from build123d import *

# Parameters (mm, degrees)
BOSS_EXTRUDE1_START                = -3.2
BOSS_EXTRUDE1_DEPTH                = 3.2
SKETCH3_R                          = 2.4
BOSS_EXTRUDE2_DEPTH                = 9.2
SKETCH4_R                          = 2.4
BOSS_EXTRUDE3_DEPTH                = 1.2
BOSS_EXTRUDE3_TAPER                = 36
CUT_EXTRUDE1_DEPTH                 = 6.925
BOSS_EXTRUDE4_DEPTH                = 3.2
TAP_DRILL_FOR_M2_2_HELICOIL1_D     = 2.3
TAP_DRILL_FOR_M2_2_HELICOIL1_DEPTH = 9.2
TAP_DRILL_FOR_M2_2_HELICOIL1_TIP   = 0.690989712


with BuildPart() as part:
    # Sketch1 → Revolve1 (revolve)
    with BuildSketch(Plane.XY):
        with BuildLine():
            Line((1.985572965, 1.6), (4.15, 1.6))
            Line((4.15, 1.6), (4.15, -1.6))
            Line((4.15, -1.6), (1.985572965, -1.6))
            ThreePointArc((1.985572965, -1.6), (2.55, 0), (1.985572965, 1.6))
        make_face()
    revolve(axis=Axis((0, 0, 0), (0, 1, 0)))

    # Sketch2 → Boss-Extrude1 (add)
    with BuildSketch(Plane(origin=(0, 1.6, 0), x_dir=(1, 0, 0), z_dir=(0, 1, 0)).offset(BOSS_EXTRUDE1_START)):
        with BuildLine():
            Line((-2.4, -6.925), (-4.001507312, -1.100199632))
            ThreePointArc((-4.001507312, -1.100199632), (0, -4.15), (4.001507312, -1.100199632))
            Line((4.001507312, -1.100199632), (2.4, -6.925))
            Line((2.4, -6.925), (2.4, -13.85))
            Line((2.4, -13.85), (-2.4, -13.85))
            Line((-2.4, -13.85), (-2.4, -6.925))
        make_face()
    extrude(amount=BOSS_EXTRUDE1_DEPTH)

    # Sketch3 → Boss-Extrude2 (add)
    with BuildSketch(Plane.XY.offset(13.85)):
        Circle(SKETCH3_R)
    extrude(amount=-BOSS_EXTRUDE2_DEPTH)

    # Sketch4 → Boss-Extrude3 (add)
    with BuildSketch(Plane(origin=(0, 0, 4.65), x_dir=(-1, 0, 0), z_dir=(0, 0, -1))):
        Circle(SKETCH4_R)
    extrude(amount=BOSS_EXTRUDE3_DEPTH, taper=BOSS_EXTRUDE3_TAPER)

    # Sketch5 → Cut-Extrude1 (cut)
    with BuildSketch(Plane.XY.offset(13.85)):
        with BuildLine():
            Line((2.4, 1.6), (1.788854382, 1.6))
            ThreePointArc((1.788854382, 1.6), (2.242013662, 0.856373015), (2.4, 0))
            Line((2.4, 0), (2.4, 1.6))
        make_face()
        with BuildLine():
            Line((2.4, -1.6), (2.4, 0))
            ThreePointArc((2.4, 0), (2.242013662, -0.856373015), (1.788854382, -1.6))
            Line((1.788854382, -1.6), (2.4, -1.6))
        make_face()
        with BuildLine():
            Line((-2.4, 1.6), (-2.4, 0))
            ThreePointArc((-2.4, 0), (-2.242013662, 0.856373015), (-1.788854382, 1.6))
            Line((-1.788854382, 1.6), (-2.4, 1.6))
        make_face()
        with BuildLine():
            Line((-2.4, 0), (-2.4, -1.6))
            Line((-2.4, -1.6), (-1.788854382, -1.6))
            ThreePointArc((-1.788854382, -1.6), (-2.242013662, -0.856373015), (-2.4, 0))
        make_face()
    extrude(amount=-CUT_EXTRUDE1_DEPTH, mode=Mode.SUBTRACT)

    # Sketch6 → Boss-Extrude4 (add)
    with BuildSketch(Plane(origin=(0, 1.6, 0), x_dir=(1, 0, 0), z_dir=(0, 1, 0))):
        Polygon((-2.4, -6.925), (-1, -12.016903392), (1, -12.016903392), (2.4, -6.925), align=None)
    extrude(amount=-BOSS_EXTRUDE4_DEPTH)

    # Tap Drill for M2.2 Helicoil1
    with Locations(Plane.XY.offset(13.85)):
        with Locations((0, 0)):
            Hole(TAP_DRILL_FOR_M2_2_HELICOIL1_D / 2, depth=TAP_DRILL_FOR_M2_2_HELICOIL1_DEPTH)
            with Locations((0, 0, -(TAP_DRILL_FOR_M2_2_HELICOIL1_DEPTH + TAP_DRILL_FOR_M2_2_HELICOIL1_TIP / 2))):  # 118° drill point
                Cone(0, TAP_DRILL_FOR_M2_2_HELICOIL1_D / 2, TAP_DRILL_FOR_M2_2_HELICOIL1_TIP, mode=Mode.SUBTRACT)


solid = part.part
Work out the finished part from the listing and answer in its coordinate system (mm). A direction names the side the tool comes from. Give positions to 0.01 mm unless a question says otherwise; leave off trailing zeros. Order: outer loops, then holes, each group sorted by start corner. A loop starts at its lowest first (then second) coordinate and runs counter-clockwise, first axis right, second up. Notation, with made-up numbers: (-0.5, -29.5) -> (52.5, -29.5) arc R31 cw to (52.5, -1.5) -> close; hole circle Ø7 at (3, 4). An arc over 180 degrees is marked (long way). Answer as a JSON object with one key per item and string values. Group by question number.
1. Section A-A on z = 10.25 is taken. Determine the outline of the cut face in (x, y).
2. Consider line 1 along Y through (x, z) = (0, 9); line 2 along Y through (x, z) = (-0.5, 7.5); line 3 along Y through (x, z) = (-2, 5.25). Determine where each line is inside the solid, lowest interval first. Write a range as [from, to].
3. Flat-ended cylindrical pins translate along their axes: pin 1 Ø1.5 at (x, z) = (2.5, 10.5) entering from +Y; pin 2 Ø2.5 at (x, z) = (2, 4.5) entering from +Y. Find the tip coordinate at first contact, or state that the pin passes through.
4. Section B-B on z = 0 is taken. Determine the outline of the cut face in (x, y), plus the area to 3 significant figures.
5. Section C-C on x = -2 is taken. Determine the outline of the cut face in (y, z), plus the area to 3 significant figures.
6. The mould has two halves that part along X. Classify faces 3 (the cylindrical face through (0.11, -0.02, -4.15)), 4 (the flat face through (-0.1, 1.6, 2.4)), 5 (the conical face through (-0.043, -0.195, 4.079)): released by +X, released by -X, zero draft, split by the parting line, or undercut.
7. A tool of negligible diameter and unlimited length cuts with its end or side. For faces 1 (the conical face through (0, 2, 4.1)), 2 (the cylindrical face through (0.91, -0.7, 9.19)), from which of +Z, -Z, +X, -X, +Y, -Y can it reach the whole face along a straight path? Write none if from no direction.
Result sheet:
{
 "1": {"outline": "circle Ø4.8 at (0, 0); hole circle Ø2.3 at (0, 0)"},
 "2": {"line 1": "y = [-2.4, -1.15], [1.15, 2.4]", "line 2": "y = [-2.35, -1.04], [1.04, 2.35]", "line 3": "y = [-1.6, 1.6]"},
 "3": {"pin 1": "stops at y = 1.64", "pin 2": "stops at y = 2.28"},
 "4": {"outline": "(-4.15, -1.6) -> (-1.99, -1.6) arc R2.55 cw to (-1.99, 1.6) -> (-4.15, 1.6) -> close; (1.99, -1.6) -> (4.15, -1.6) -> (4.15, 1.6) -> (1.99, 1.6) arc R2.55 cw to start", "area": "11.4 mm^2"},
 "5": {"outline": "(-1.6, -3.64) -> (1.6, -3.64) -> (1.6, 8.38) -> (1.33, 8.38) -> (1.33, 13.85) -> (-1.33, 13.85) -> (-1.33, 8.38) -> (-1.6, 8.38) -> close; hole circle Ø3.16 at (0, 0)", "area": "45.1 mm^2"},
 "6": {"face 3": "split by the parting line", "face 4": "zero draft", "face 5": "undercut"},
 "7": {"face 1": "-Z, +Y", "face 2": "+Z"}
}
